```python
from build123d import *

# Parameters (mm, degrees)
SKETCH1_W           = 100.584
SKETCH1_H           = 75.184
BOSS_EXTRUDE1_DEPTH = 2.54
SKETCH2_W           = 100.584
SKETCH2_H           = 75.184
SKETCH2_W_2         = 95.758
SKETCH2_H_2         = 70.358
BOSS_EXTRUDE2_DEPTH = 35.56
SKETCH3_W           = 19.05
SKETCH3_H           = 7.62
CUT_EXTRUDE1_DEPTH  = 132.230274373
FILLET1_R           = 3.81
CUT_EXTRUDE2_DEPTH  = 6.35
SKETCH5_W           = 15.278664452
SKETCH5_H           = 26.67
CUT_EXTRUDE3_DEPTH  = 6.35
SKETCH6_W           = 11.43
SKETCH6_H           = 21.859082526
CUT_EXTRUDE4_DEPTH  = 6.35


with BuildPart() as part:
    # Sketch1 → Boss-Extrude1 (new body)
    with BuildSketch(Plane(origin=(0, 0, 0), x_dir=(1, 0, 0), z_dir=(0, 1, 0))):
        with Locations((50.292, 37.592)):
            Rectangle(SKETCH1_W, SKETCH1_H)
    extrude(amount=BOSS_EXTRUDE1_DEPTH)

    # Sketch2 → Boss-Extrude2 (add)
    with BuildSketch(Plane(origin=(0, 2.54, 0), x_dir=(1, 0, 0), z_dir=(0, 1, 0))):
        with Locations((50.292, 37.592)):
            Rectangle(SKETCH2_W, SKETCH2_H)
        with Locations((50.292, 37.592)):
            Rectangle(SKETCH2_W_2, SKETCH2_H_2, mode=Mode.SUBTRACT)
    extrude(amount=BOSS_EXTRUDE2_DEPTH)

    # Sketch3 → Cut-Extrude1 (cut, through all)
    with BuildSketch(Plane(origin=(0, 0, -75.184), x_dir=(-1, 0, 0), z_dir=(0, 0, -1))):
        with Locations((-50.292, 34.29)):
            Rectangle(SKETCH3_W, SKETCH3_H)
    extrude(amount=-CUT_EXTRUDE1_DEPTH, mode=Mode.SUBTRACT)

    # Fillet1
    fillet1_edges = [part.edges().sort_by_distance(p)[0] for p in [
        (40.767, 30.48, -1.2065),
        (59.817, 30.48, -1.2065),
        (59.817, 30.48, -73.9775),
        (40.767, 30.48, -73.9775),
    ]]
    fillet(fillet1_edges, radius=FILLET1_R)
    fillet1_2_edges = [part.edges().sort_by_distance(p)[0] for p in [
        (40.767, 38.1, -1.2065),
        (59.817, 38.1, -1.2065),
        (59.817, 38.1, -73.9775),
        (40.767, 38.1, -73.9775),
    ]]
    fillet(fillet1_2_edges, radius=FILLET1_R - 0.0001)  # a hair under: the kernel refuses the full size

    # Sketch4 → Cut-Extrude2 (cut)
    with BuildSketch(Plane.ZY):
        Polygon((-21.270705039, 38.1), (-58.928, 38.1), (-65.278, 38.1), (-65.278, 31.750254), (-65.278, 27.940254), (-58.928, 27.940254), (-21.270705039, 27.940254), align=None)
    extrude(amount=-CUT_EXTRUDE2_DEPTH, mode=Mode.SUBTRACT)

    # Sketch5 → Cut-Extrude3 (cut)
    with BuildSketch(Plane(origin=(100.584, 0, 0), x_dir=(0, 0, -1), z_dir=(1, 0, 0))):
        with Locations((16.998667774, 24.765254)):
            Rectangle(SKETCH5_W, SKETCH5_H)
    extrude(amount=-CUT_EXTRUDE3_DEPTH, mode=Mode.SUBTRACT)

    # Sketch6 → Cut-Extrude4 (cut)
    with BuildSketch(Plane(origin=(0, 0, -75.184), x_dir=(-1, 0, 0), z_dir=(0, 0, -1))):
        with Locations((-50.292, 19.550458737)):
            Rectangle(SKETCH6_W, SKETCH6_H)
    extrude(amount=-CUT_EXTRUDE4_DEPTH, mode=Mode.SUBTRACT)


solid = part.part
```
CAD build for the part. Positions are in the model's coordinates, mm. A direction names the side the tool comes from. Round coordinates to 2 decimals unless told otherwise and drop trailing zeros. Write each loop counter-clockwise with the first axis right and the second up, starting at its lowest first coordinate (ties: lowest second). Pieces come first, ordered by that corner, then holes. Notation, with made-up numbers: (79.5, -22) -> (83.5, -22) arc R21 cw to (83.5, 13) -> close; hole circle Ø4 at (28.25, 69). An arc over 180 degrees is marked (long way). Answer in a Markdown table with one row per item. Add a question column.
Item 1: Drill centre lines: line 1 (X direction, y = 36, z = -6); line 2 (Z direction, x = 86, y = 5.5); line 3 (Y direction, x = 61.5, z = -6). Where is each one in solid material? Low to high. Write a range as from..to.
Item 2: Saw through at A-A, the plane y = 17.5. Write the cut outline in (x, z).
Item 3: Drop flat-ended pins along their axis: pin 1 Ø1 at (y, z) = (28.5, -45) entering from -X; pin 2 Ø1.9 at (x, z) = (0.5, -52.5) entering from +Y; pin 3 Ø2.5 at (x, z) = (51, -74) entering from +Y. Give the stop position or say it passes through.
Item 4: Which spindle directions (+Z, -Z, +X, -X, +Y, -Y) get a long thin tool onto all of the face, cutting with end or side? Do faces 1 (the face through (56.007, 19, -74)), 2 (the face through (60.96, 37.01, -1.19)), 3 (the face through (99, 25, -24.638)). Say none if no direction does.
Item 5: Mould opens along Z. For faces 4 (the face through (61, 19, -75.184)), 5 (the face through (39, 20, -72.771)), 6 (the face through (50, 0, -38)), 7 (the face through (1, 27.94, -44)) say: pulls with the +Z half, pulls with the -Z half, needs draft (parallel to the pull), parting line crosses it, or undercut.
Item 6: Saw through at B-B, the plane x = 52. Write the cut outline in (y, z), then the cut area to 3 significant figures.
Item 7: Saw through at C-C, the plane z = -22.5. Write the cut outline in (x, y), then the cut area to 3 significant figures.
Findings below:
| question | item | result |
|---|---|---|
| 1 | line 1 | x = 0..2.41, 98.17..100.58 |
| 1 | line 2 | z = -75.18..-72.77, -2.41..0 |
| 1 | line 3 | y = 0..2.54 |
| 2 | outline | (0, -75.18) -> (44.58, -75.18) -> (44.58, -72.77) -> (2.41, -72.77) -> (2.41, -2.41) -> (98.17, -2.41) -> (98.17, -9.36) -> (100.58, -9.36) -> (100.58, 0) -> (0, 0) -> close; (56.01, -75.18) -> (100.58, -75.18) -> (100.58, -24.64) -> (98.17, -24.64) -> (98.17, -72.77) -> (56.01, -72.77) -> close |
| 3 | pin 1 | stops at x = 98.17 |
| 3 | pin 2 | stops at y = 27.94 |
| 3 | pin 3 | stops at y = 8.62 |
| 4 | face 1 | -Z, +Y |
| 4 | face 2 | +Z, -Z, +Y |
| 4 | face 3 | +X, +Y |
| 5 | face 4 | pulls with the -Z half |
| 5 | face 5 | undercut |
| 5 | face 6 | needs draft |
| 5 | face 7 | undercut |
| 6 | outline | (0, -75.18) -> (8.62, -75.18) -> (8.62, -72.77) -> (2.54, -72.77) -> (2.54, -2.41) -> (30.48, -2.41) -> (30.48, 0) -> (0, 0) -> close |
| 6 | area | 273 mm^2 |
| 7 | outline | (0, 0) -> (100.58, 0) -> (100.58, 11.43) -> (98.17, 11.43) -> (98.17, 2.54) -> (2.41, 2.54) -> (2.41, 27.94) -> (0, 27.94) -> close |
| 7 | area | 338 mm^2 |
